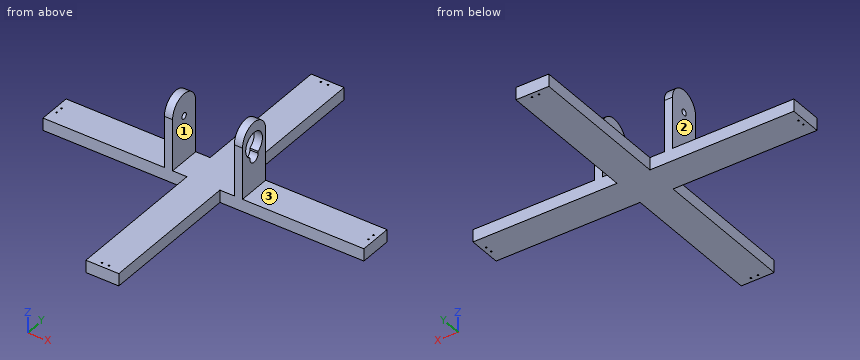
from build123d import *

# Parameters (mm, degrees)
Y_KSEKLIK_EKSTR_ZYON1_DEPTH = 3
IZIM2_R                     = 0.35
KES_EKSTR_ZYON1_DEPTH       = 5
IZIM3_W                     = 4
IZIM3_H                     = 16
Y_KSEKLIK_EKSTR_ZYON4_DEPTH = 36
KES_EKSTR_ZYON2_DEPTH       = 122.556571192
KES_EKSTR_ZYON2_DEPTH_BACK  = 122.556571192
KES_EKSTR_ZYON3_DEPTH       = 100
IZIM8_R                     = 1.5
KES_EKSTR_ZYON4_DEPTH       = 30


with BuildPart() as part:
    # Çizim1 → Yükseklik-Ekstrüzyon1 (new, symmetric)
    with BuildSketch(Plane.XY):
        Polygon((8, 70), (-8, 70), (-8, 0), (-78, 0), (-78, -16), (-8, -16), (-8, -86), (8, -86), (8, -16), (78, -16), (78, 0), (8, 0), align=None)
    extrude(amount=Y_KSEKLIK_EKSTR_ZYON1_DEPTH, both=True)

    # Çizim2 → Kes-Ekstrüzyon1 (cut, symmetric)
    with BuildSketch(Plane.XY):
        with Locations(Location((-75.8, -6.3, 0), (0, 0, 180))):
            Circle(IZIM2_R)
        with Locations(Location((-75.8, -9.7, 0), (0, 0, 180))):
            Circle(IZIM2_R)
        with Locations(Location((-1.7, 67.8, 0), (0, 0, 180))):
            Circle(IZIM2_R)
        with Locations(Location((1.7, 67.8, 0), (0, 0, 180))):
            Circle(IZIM2_R)
        with Locations(Location((75.804898835, -6.19877905, 0), (0, 0, 180))):
            Circle(IZIM2_R)
        with Locations(Location((75.804898835, -9.59877905, 0), (0, 0, 180))):
            Circle(IZIM2_R)
        with Locations((-75.804898835, 141.79877905)):
            Circle(IZIM2_R)
        with Locations((-75.804898835, 145.19877905)):
            Circle(IZIM2_R)
        with Locations((73.99877905, 143.604898835)):
            Circle(IZIM2_R)
        with Locations((77.39877905, 143.604898835)):
            Circle(IZIM2_R)
        with Locations(Location((-1.7, -83.8, 0), (0, 0, 180))):
            Circle(IZIM2_R)
        with Locations(Location((1.7, -83.8, 0), (0, 0, 180))):
            Circle(IZIM2_R)
    extrude(amount=KES_EKSTR_ZYON1_DEPTH, both=True, mode=Mode.SUBTRACT)

    # Çizim3 → Yükseklik-Ekstrüzyon4 (add)
    with BuildSketch(Plane.XY):
        with Locations((-17, -8)):
            Rectangle(IZIM3_W, IZIM3_H)
        with Locations((17, -8)):
            Rectangle(IZIM3_W, IZIM3_H)
    extrude(amount=Y_KSEKLIK_EKSTR_ZYON4_DEPTH)

    # Çizim6 → Kes-Ekstrüzyon2 (cut, two sides: drawn at the far end of the back side and taken through both)
    with BuildSketch(Plane(origin=(0, 0, 0), x_dir=(0, 0, -1), z_dir=(1, 0, 0)).offset(-KES_EKSTR_ZYON2_DEPTH_BACK)):
        with BuildLine():
            Line((-36, 0), (-39.977521608, 0))
            Line((-39.977521608, 0), (-39.977521608, -16))
            Line((-39.977521608, -16), (-36, -16))
            Line((-36, -16), (-28, -16))
            ThreePointArc((-28, -16), (-36, -8), (-28, 0))
            Line((-28, 0), (-36, 0))
        make_face()
    extrude(amount=KES_EKSTR_ZYON2_DEPTH + KES_EKSTR_ZYON2_DEPTH_BACK, mode=Mode.SUBTRACT)

    # Çizim7 → Kes-Ekstrüzyon3 (cut)
    with BuildSketch(Plane(origin=(0, 0, 0), x_dir=(0, 0, -1), z_dir=(1, 0, 0))):
        with BuildLine():
            Line((-19.2, -5.2), (-20.12062996, -5.2))
            ThreePointArc((-20.12062996, -5.2), (-31, -8), (-20.12062996, -10.8))
            Line((-20.12062996, -10.8), (-19.2, -10.8))
            ThreePointArc((-19.2, -10.8), (-16.4, -8), (-19.2, -5.2))
        make_face()
    extrude(amount=KES_EKSTR_ZYON3_DEPTH, mode=Mode.SUBTRACT)

    # Çizim8 → Kes-Ekstrüzyon4 (cut)
    with BuildSketch(Plane(origin=(-9.5, 0, 0), x_dir=(0, 0, -1), z_dir=(1, 0, 0))):
        with Locations((-25.2, -8)):
            Circle(IZIM8_R)
    extrude(amount=-KES_EKSTR_ZYON4_DEPTH, mode=Mode.SUBTRACT)


solid = part.part
The model under review builds one solid part; all positions refer to its coordinate system, in mm. Face numbers are marked on the shaded views. A direction names the side the tool comes from. Give positions to 0.01 mm unless a question says otherwise; leave off trailing zeros. Write each loop counter-clockwise with the first axis right and the second up, starting at its lowest first coordinate (ties: lowest second). Pieces come first, ordered by that corner, then holes.
1. Wall thickness on L1, parallel to X at y = 67.8, z = -1.35; L2, parallel to Y at x = 1.7, z = -1.6; L3, parallel to Y at x = -15.85, z = 25.2: over which ranges is each line inside the solid? List them lowest first.
2. Add section A-A, the plane z = 12. Write out the cut boundary in (x, y), plus the area to 3 significant figures.
3. Tool access review of the marked faces 1, 2 and 3: name each direction out of +Z, -Z, +X, -X, +Y, -Y from which nothing blocks a thin tool from reaching the whole face with its end or side.
4. For P1, Ø9.5, axis at y = -8, z = 25.2, coming from the +X side; P2, Ø1.5, axis at x = 5.5, y = -69, coming from the +Z side; P3, Ø17.5, axis at y = -5, z = 21.5, coming from the -X side, all flat-tipped, find the tip position at first contact; note any pin that passes through.
5. Add section C-C, the plane x = 12. Write out the cut boundary in (y, z).
6. Add section B-B, the plane y = 14. Write out the cut boundary in (x, z).
Worked answers:
1. L1: x = -8 to -2.05, -1.35 to 1.35, 2.05 to 8
1. L2: y = -86 to -84.15, -83.45 to 67.45, 68.15 to 70
1. L3: y = -16 to -9.5, -6.5 to 0
2. outline: (-19, -16) - (-15, -16) - (-15, 0) - (-19, 0) - close; (15, -16) - (19, -16) - (19, 0) - (15, 0) - close
2. area: 128 mm2
3. face 1: +Z, +Y, -Y
3. face 2: +Z, -X, +Y, -Y
3. face 3: +Z, +X, +Y, -Y
4. P1: stops at x = -15
4. P2: stops at z = 3
4. P3: stops at x = -19
5. outline: (-16, -3) - (0, -3) - (0, 3) - (-16, 3) - close
6. outline: (-8, -3) - (8, -3) - (8, 3) - (-8, 3) - close
